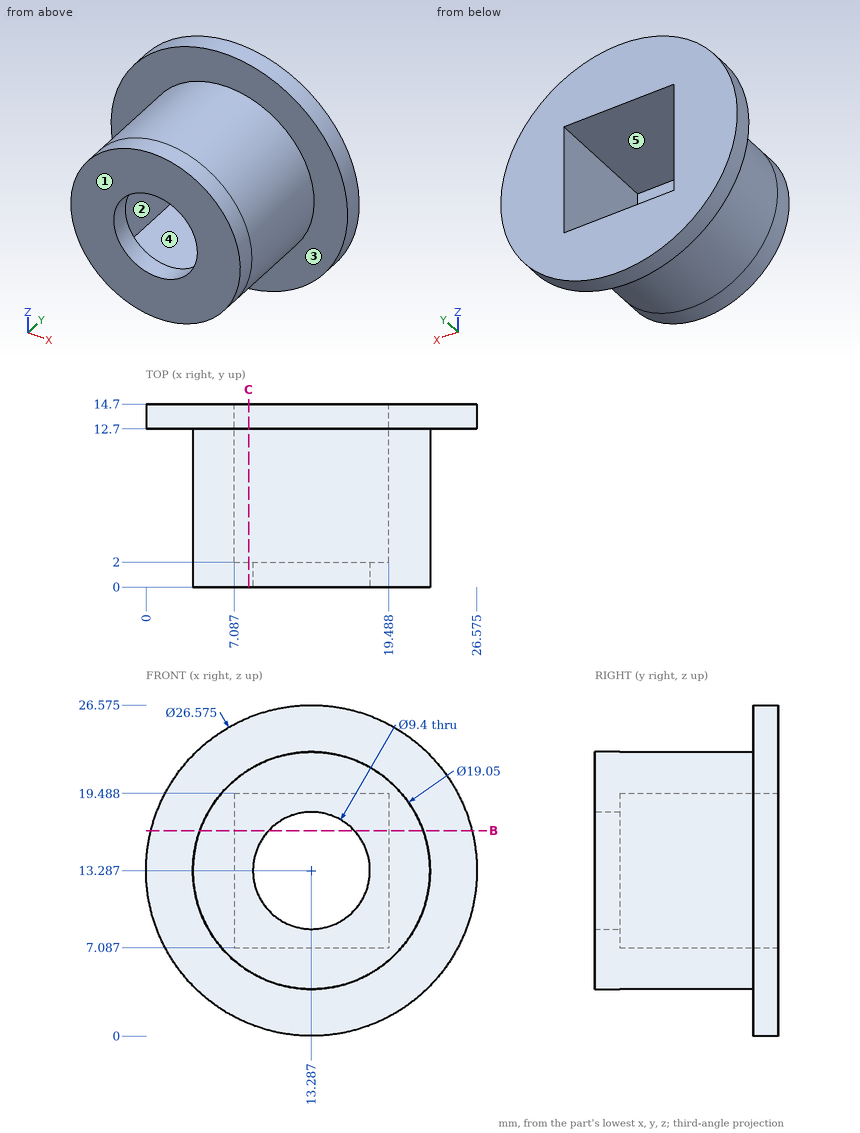
Job drawing, mm, ordinate dimensions from the low corner. One solid piece. A direction names the side the tool comes from. Give positions to 0.01 mm unless a question says otherwise; leave off trailing zeros. Loops run counter-clockwise (first coordinate to the right, second up) from the corner with the lowest first, then second, coordinate; pieces in that order, holes last. Notation, with made-up numbers: M 79.5,26 L 127.5,26 A31 cw 127.5,50 Z; hole C -36.75,41.5 d9. An arc over 180 degrees is marked long. Use one line per item in the form item = value.
Item 1: Two-plate mould, pull along X, no slides. Class the marked faces 3, 4 and 5: released by +X, released by -X, zero draft, split by the parting line, or undercut.
Filled in:
face_3 = zero draft
face_4 = undercut
face_5 = undercut
Item 2: Slice it at B-B on z = 16.5. List the corners of the cut face in (x, y) (1 decimal).
Filled in:
outline = M 0.4,12.7 L 4.3,12.7 L 4.3,0 L 9.9,0 L 9.9,2 L 7.1,2 L 7.1,14.7 L 0.4,14.7 Z; M 16.7,0 L 22.3,0 L 22.3,12.7 L 26.2,12.7 L 26.2,14.7 L 19.5,14.7 L 19.5,2 L 16.7,2 Z
Item 3: Flat gauge pins, fed straight in: pin 1 Ø2 at (x, y) = (4, 12) entering from +Z; pin 2 Ø1 at (x, y) = (15, 12.5) entering from +Z (1 decimal); pin 3 Ø6 at (y, z) = (8, 16) entering from +X; pin 4 Ø6 at (x, z) = (14, 14.5) entering from +Y. Where does each tip first touch, or does it go through?
Filled in:
pin_1 = 23.44
pin_2 = 26.5
pin_3 = 22.81
pin_4 = through
Item 4: Drill centre lines: L1, parallel to Z at x = 13.5, y = 11.75 (1 decimal); L2, parallel to Y at x = 19.25, z = 21; L3, parallel to Y at x = 19, z = 17. Where is each one in solid material? Low to high.
Filled in:
L1 = 3.8 to 7.1, 19.5 to 22.8
L2 = 12.7 to 14.7
L3 = 0 to 2
Item 5: Which spindle directions (+Z, -Z, +X, -X, +Y, -Y) get a long thin tool onto all of the face, cutting with end or side? Do the marked faces 1 and 2. Say none if no direction does.
Filled in:
face_1 = +Z, -Z, +X, -X, -Y
face_2 = +Y
Item 6: Slice it at C-C on x = 8.25. List the corners of the cut face in (y, z).
Filled in:
outline = M 0,5.2 L 12.7,5.2 L 12.7,0.99 L 14.7,0.99 L 14.7,7.09 L 2,7.09 L 2,19.49 L 14.7,19.49 L 14.7,25.58 L 12.7,25.58 L 12.7,21.37 L 0,21.37 Z
